from build123d import *

# Parameters (mm, degrees)
F0_W      = 150
F0_H      = 200
F1_DEPTH  = 5
F2_W      = 15
F2_H      = 5
F3_DEPTH  = 190
F4_W      = 15
F4_H      = 5
F5_DEPTH  = 170
F7_DEPTH  = 5
F9_W      = 120
F9_H      = 170
F10_DEPTH = 25


with BuildPart() as f1:
    # F0 (on Front) → F1 (new body)
    with BuildSketch(Plane.XZ):
        Rectangle(F0_W, F0_H)
    extrude(amount=F1_DEPTH)

    # F2 (on face) → F3 (join)
    with BuildSketch(Plane.XZ.offset(5)):
        with Locations((67.5, 97.5)):
            Rectangle(F2_W, F2_H)
        with Locations((67.5, -97.5)):
            Rectangle(F2_W, F2_H)
    extrude(amount=F3_DEPTH)

    # F4 (on face) → F5 (join)
    with BuildSketch(Plane.XZ.offset(5)):
        with Locations((-67.5, 97.5)):
            Rectangle(F4_W, F4_H)
        with Locations((-67.5, -97.5)):
            Rectangle(F4_W, F4_H)
    extrude(amount=F5_DEPTH)

    # F6 (on face) → F7 (join)
    with BuildSketch(Plane.XY.offset(100)):
        Polygon((-60, -160), (-60, -175), (60, -195), (60, -180), align=None)
    extrude(amount=-F7_DEPTH)

    # F8: F1 across plane


with BuildPart() as f1_1:
    add(f1.part)
    add(f1.part.mirror(Plane.XY))

    # F9 (on face) → F10 (cut)
    with BuildSketch(Plane.XZ.offset(5)):
        Rectangle(F9_W, F9_H)
    extrude(amount=-F10_DEPTH, mode=Mode.SUBTRACT)


solid = f1_1.part
Design review of the part built by this model. Coordinates are the model's own, in mm. A direction names the side the tool comes from. Coordinates: 2 decimals unless noted, no trailing zeros. Order: outer loops, then holes, each group sorted by start corner. A loop starts at its lowest first (then second) coordinate and runs counter-clockwise, first axis right, second up.
Item 1: For line 1 (Z direction, x = -62, y = -108.5); line 2 (Y direction, x = -68, z = 19.5), list the stretches that pass through material, from the lowest coordinate up.
Item 2: Take a section at A-A, the plane y = -26. Write out the cut boundary in (x, z).
Item 3: The part is to be moulded in two halves that separate along Z. For faces 5 (the flat face through (61, -97, 100)), 6 (the flat face through (60, -3, -1)), 7 (the flat face through (60, -91, -98)), 8 (the flat face through (-11, -170, 95)), say which applies: pulls with the +Z half, pulls with the -Z half, needs draft (parallel to the pull), parting line crosses it, or undercut.
Item 4: Take a section at C-C, the plane x = 8. Write out the cut boundary in (y, z), then the cut area to 3 significant figures.
Item 5: For faces 1 (the flat face through (0.84, -170.14, 97.54)), 2 (the flat face through (67, -195, 98)), 3 (the flat face through (-1, -3, 85)), 4 (the flat face through (-68, -175, -97)), list the 3-axis set-ups (+Z, -Z, +X, -X, +Y, -Y) from which the entire face can be reached by the end or side of a thin tool; tool diameter is ignored.
Item 6: For pin 1 Ø2 at (x, z) = (59.5, -38) entering from +Y; pin 2 Ø4 at (x, z) = (-70, -98) entering from -Y, all flat-tipped, find the tip position at first contact; note any pin that passes through.
Item 7: Take a section at B-B, the plane z = -32. Write out the cut boundary in (x, y).
The answers:
1. line 1: z = -100 to -95, 95 to 100
1. line 2: y = -5 to 0
2. outline: (-75, -100) - (-60, -100) - (-60, -95) - (-75, -95) - close; (-75, 95) - (-60, 95) - (-60, 100) - (-75, 100) - close; (60, -100) - (75, -100) - (75, -95) - (60, -95) - close; (60, 95) - (75, 95) - (75, 100) - (60, 100) - close
3. face 5: pulls with the +Z half
3. face 6: undercut
3. face 7: needs draft
3. face 8: undercut
4. outline: (-186.33, -100) - (-171.33, -100) - (-171.33, -95) - (-186.33, -95) - close; (-186.33, 95) - (-171.33, 95) - (-171.33, 100) - (-186.33, 100) - close; (-5, -100) - (0, -100) - (0, -85) - (-5, -85) - close; (-5, 85) - (0, 85) - (0, 100) - (-5, 100) - close
4. area: 300 mm2
5. face 1: +Z, -Z
5. face 2: +Z, -Z, +X, -X, -Y
5. face 3: +Y, -Y
5. face 4: +Z, -Z, -X, -Y
6. pin 1: stops at y = 0
6. pin 2: stops at y = -175
7. outline: (-75, -5) - (-60, -5) - (-60, 0) - (-75, 0) - close; (60, -5) - (75, -5) - (75, 0) - (60, 0) - close
